CAD build for the part. Positions are in the model's coordinates, mm. A direction names the side the tool comes from. Give positions to 0.01 mm unless a question says otherwise; leave off trailing zeros. Loops run counter-clockwise (first coordinate to the right, second up) from the corner with the lowest first, then second, coordinate; pieces in that order, holes last. Notation, with made-up numbers: M -39.75,-20 L -17.75,-20 A15 cw -17.75,-9 Z; hole C 19,66.25 d10. An arc over 180 degrees is marked long. Answer as CSV lines item,"result".
from build123d import *

# Parameters (mm, degrees)
SKETCH_1_W          = 11
SKETCH_1_H          = 9.5
EXTRUDE_1_DEPTH     = 3
CUT_EXTRUDE_1_DEPTH = 0.5
FILLET_1_R          = 0.7
SKETCH_3_R          = 1.9
EXTRUDE_2_DEPTH     = 0.2
CUT_EXTRUDE_2_DEPTH = 15.783098457
EXTRUDE_3_DEPTH     = 0.2
EXTRUDE_4_DEPTH     = 1
SKETCH_7_R          = 0.75
EXTRUDE_5_DEPTH     = 0.5
SKETCH_8_R          = 0.75
SKETCH_8_R_2        = 2
EXTRUDE_6_DEPTH     = 0.3


with BuildPart() as part:
    # 草图1 → 凸台-拉伸1 (new body)
    with BuildSketch(Plane.XY):
        with Locations((5.5, 4.75)):
            Rectangle(SKETCH_1_W, SKETCH_1_H)
    extrude(amount=EXTRUDE_1_DEPTH)

    # 草图2 → 切除-拉伸1 (cut)
    with BuildSketch(Plane.XY.offset(3)):
        with BuildLine():
            Line((9.028427125, 5.75), (10.33067791, 5.75))
            ThreePointArc((10.33067791, 5.75), (9.020226339, 7.929437592), (6.7, 8.970485754))
            Line((6.7, 8.970485754), (6.7, 7.708039892))
            ThreePointArc((6.7, 7.708039892), (8.130825429, 7.046064713), (9.028427125, 5.75))
        make_face()
        with BuildLine():
            Line((3.371572875, 3.75), (2.06932209, 3.75))
            ThreePointArc((2.06932209, 3.75), (3.379773661, 1.570562408), (5.7, 0.529514246))
            Line((5.7, 0.529514246), (5.7, 1.791960108))
            ThreePointArc((5.7, 1.791960108), (4.269174571, 2.453935287), (3.371572875, 3.75))
        make_face()
        with BuildLine():
            Line((2.06932209, 5.75), (3.371572875, 5.75))
            ThreePointArc((3.371572875, 5.75), (4.269174571, 7.046064713), (5.7, 7.708039892))
            Line((5.7, 7.708039892), (5.7, 8.970485754))
            ThreePointArc((5.7, 8.970485754), (3.379773661, 7.929437592), (2.06932209, 5.75))
        make_face()
        with BuildLine():
            Line((10.33067791, 3.75), (9.028427125, 3.75))
            ThreePointArc((9.028427125, 3.75), (8.130825429, 2.453935287), (6.7, 1.791960108))
            Line((6.7, 1.791960108), (6.7, 0.529514246))
            ThreePointArc((6.7, 0.529514246), (9.020226339, 1.570562408), (10.33067791, 3.75))
        make_face()
        with BuildLine():
            Line((5.7, 7.199489743), (5.7, 6.95))
            Line((5.7, 6.95), (6.7, 6.95))
            Line((6.7, 6.95), (6.7, 7.199489743))
            ThreePointArc((6.7, 7.199489743), (8.7, 4.75), (6.7, 2.300510257))
            Line((6.7, 2.300510257), (6.7, 2.55))
            Line((6.7, 2.55), (5.7, 2.55))
            Line((5.7, 2.55), (5.7, 2.300510257))
            ThreePointArc((5.7, 2.300510257), (3.7, 4.75), (5.7, 7.199489743))
        make_face()
    extrude(amount=-CUT_EXTRUDE_1_DEPTH, mode=Mode.SUBTRACT)

    # 圆角1
    fillet_1_edges = [part.edges().sort_by_distance(p)[0] for p in [
        (0, 0, 1.5),
        (0, 9.5, 1.5),
        (11, 9.5, 1.5),
        (11, 0, 1.5),
    ]]
    fillet(fillet_1_edges, radius=FILLET_1_R)

    # 草图3 → 凸台-拉伸2 (add)
    with BuildSketch(Plane.XY.offset(2.5)):
        with Locations((6.2, 4.75)):
            Circle(SKETCH_3_R)
    extrude(amount=EXTRUDE_2_DEPTH)

    # 草图4 → 切除-拉伸2 (cut, through all)
    with BuildSketch(Plane.XY.offset(2.7)):
        Polygon((6.15, 5.55), (6.25, 5.55), (6.25, 5.25), (7.3, 5.25), (7.3, 4.25), (6.25, 4.25), (6.25, 3.95), (6.15, 3.95), (6.15, 4.25), (5.1, 4.25), (5.1, 4.75), (5.1, 5.25), (6.15, 5.25), align=None)
    extrude(amount=-CUT_EXTRUDE_2_DEPTH, mode=Mode.SUBTRACT)

    # 草图5 → 凸台-拉伸3 (add)
    with BuildSketch(Plane.XY.offset(2.7)):
        with BuildLine():
            Line((5.1, 4.25), (5.1, 5.25))
            Line((5.1, 5.25), (4.366969722, 5.25))
            ThreePointArc((4.366969722, 5.25), (4.3, 4.75), (4.366969722, 4.25))
            Line((4.366969722, 4.25), (5.1, 4.25))
        make_face()
        with BuildLine():
            Line((7.3, 5.25), (8.033030278, 5.25))
            ThreePointArc((8.033030278, 5.25), (8.1, 4.75), (8.033030278, 4.25))
            Line((8.033030278, 4.25), (7.3, 4.25))
            Line((7.3, 4.25), (7.3, 5.25))
        make_face()
    extrude(amount=EXTRUDE_3_DEPTH)

    # 草图6 → 凸台-拉伸4 (add)
    with BuildSketch(Plane.XZ.offset(-4.25)):
        Polygon((5.1, 2.9), (5.1, 3.2), (4.1, 2.9), align=None)
        Polygon((7.3, 2.9), (7.3, 3.2), (8.3, 2.9), align=None)
    extrude(amount=-EXTRUDE_4_DEPTH)

    # 草图7 → 凸台-拉伸5 (add)
    with BuildSketch(Plane(origin=(0, 0, 0), x_dir=(-1, 0, 0), z_dir=(0, 0, -1))):
        with Locations((-10, 8.5)):
            Circle(SKETCH_7_R)
        with Locations((-3, 8.5)):
            Circle(SKETCH_7_R)
        with Locations((-3, 1)):
            Circle(SKETCH_7_R)
        with Locations((-10, 1)):
            Circle(SKETCH_7_R)
    extrude(amount=EXTRUDE_5_DEPTH)

    # 草图8 → 凸台-拉伸6 (add)
    with BuildSketch(Plane(origin=(0, 0, 0), x_dir=(-1, 0, 0), z_dir=(0, 0, -1))):
        with BuildLine():
            Line((-2.05, 0.7), (-2.05, 2.75))
            Line((-2.05, 2.75), (-2.55, 2.75))
            Line((-2.55, 2.75), (-2.55, 4.75))
            Line((-2.55, 4.75), (-2.55, 6.75))
            Line((-2.55, 6.75), (-2.05, 6.75))
            Line((-2.05, 6.75), (-2.05, 8.8))
            ThreePointArc((-2.05, 8.8), (-2.240380592, 9.259619408), (-2.7, 9.45))
            Line((-2.7, 9.45), (-4.5, 9.45))
            Line((-4.5, 9.45), (-4.5, 8.95))
            Line((-4.5, 8.95), (-6.5, 8.95))
            Line((-6.5, 8.95), (-8.5, 8.95))
            Line((-8.5, 8.95), (-8.5, 9.45))
            Line((-8.5, 9.45), (-10.3, 9.45))
            ThreePointArc((-10.3, 9.45), (-10.759619408, 9.259619408), (-10.95, 8.8))
            Line((-10.95, 8.8), (-10.95, 6.75))
            Line((-10.95, 6.75), (-10.45, 6.75))
            Line((-10.45, 6.75), (-10.45, 4.75))
            Line((-10.45, 4.75), (-10.45, 2.75))
            Line((-10.45, 2.75), (-10.95, 2.75))
            Line((-10.95, 2.75), (-10.95, 0.7))
            ThreePointArc((-10.95, 0.7), (-10.759619408, 0.240380592), (-10.3, 0.05))
            Line((-10.3, 0.05), (-8.5, 0.05))
            Line((-8.5, 0.05), (-8.5, 0.55))
            Line((-8.5, 0.55), (-7.5, 0.55))
            Line((-7.5, 0.55), (-6.5, 0.55))
            Line((-6.5, 0.55), (-4.5, 0.55))
            Line((-4.5, 0.55), (-4.5, 0.05))
            Line((-4.5, 0.05), (-2.7, 0.05))
            ThreePointArc((-2.7, 0.05), (-2.240380592, 0.240380592), (-2.05, 0.7))
        make_face()
        with Locations(Location((-10, 8.5, 0), (0, 0, 180))):
            Circle(SKETCH_8_R, mode=Mode.SUBTRACT)
        with Locations(Location((-3, 8.5, 0), (0, 0, 180))):
            Circle(SKETCH_8_R, mode=Mode.SUBTRACT)
        with Locations(Location((-10, 1, 0), (0, 0, 180))):
            Circle(SKETCH_8_R, mode=Mode.SUBTRACT)
        with Locations(Location((-3, 1, 0), (0, 0, 180))):
            Circle(SKETCH_8_R, mode=Mode.SUBTRACT)
        with Locations((-6.2, 4.75)):
            Circle(SKETCH_8_R_2, mode=Mode.SUBTRACT)
    extrude(amount=EXTRUDE_6_DEPTH)


solid = part.part
1) Band-saw the part on B-B on z = 0.9. Give the cut face in (x, y).
Answer below:
outline,"M 0,0.7 A0.7 ccw 0.7,0 L 10.3,0 A0.7 ccw 11,0.7 L 11,8.8 A0.7 ccw 10.3,9.5 L 0.7,9.5 A0.7 ccw 0,8.8 Z; hole M 5.1,4.25 L 6.15,4.25 L 6.15,3.95 L 6.25,3.95 L 6.25,4.25 L 7.3,4.25 L 7.3,5.25 L 6.25,5.25 L 6.25,5.55 L 6.15,5.55 L 6.15,5.25 L 5.1,5.25 Z"
2) Flat gauge pins, fed straight in: pin 1 (1 mm diameter, centred on x = 4.5, y = 2, fed in from +Z); pin 2 (4.5 mm diameter, centred on x = 8, y = 5, fed in from -Z). Where does each tip first touch, or does it go through?
Answer below:
pin 1,"stops at z = 3"
pin 2,"stops at z = -0.3"
3) Band-saw the part on D-D on x = 3. Give the cut face in (y, z).
Answer below:
outline,"M 0,0 L 0.05,0 L 0.05,-0.3 L 0.25,-0.3 L 0.25,-0.5 L 1.75,-0.5 L 1.75,-0.3 L 7.75,-0.3 L 7.75,-0.5 L 9.25,-0.5 L 9.25,-0.3 L 9.45,-0.3 L 9.45,0 L 9.5,0 L 9.5,3 L 7.55,3 L 7.55,2.5 L 5.75,2.5 L 5.75,3 L 3.75,3 L 3.75,2.5 L 1.95,2.5 L 1.95,3 L 0,3 Z"
4) Which spindle directions (+Z, -Z, +X, -X, +Y, -Y) get a long thin tool onto all of the face, cutting with end or side? Do faces 4 (the face through (6, 4, 0)), 5 (the face through (6, 4, 2.7)), 6 (the face through (5.1, 5, 2)). Say none if no direction does.
Answer below:
face 4,"-Z"
face 5,"+Z"
face 6,"+Z, -Z"
5) Band-saw the part on C-C on y = 8.5. Give the cut face in (x, z), and give its area (3 significant figures).
Answer below:
outline,"M 0,0 L 2.05,0 L 2.05,-0.3 L 2.25,-0.3 L 2.25,-0.5 L 3.75,-0.5 L 3.75,-0.3 L 9.25,-0.3 L 9.25,-0.5 L 10.75,-0.5 L 10.75,-0.3 L 10.95,-0.3 L 10.95,0 L 11,0 L 11,3 L 8.2,3 L 8.2,2.5 L 6.7,2.5 L 6.7,3 L 5.7,3 L 5.7,2.5 L 4.2,2.5 L 4.2,3 L 0,3 Z"
area,"34.8 mm^2"
6) Band-saw the part on A-A on y = 4.75. Give the cut face in (x, z), and give its area (3 significant figures).
Answer below:
outline,"M 0,0 L 2.55,0 L 2.55,-0.3 L 4.2,-0.3 L 4.2,0 L 5.1,0 L 5.1,3.2 L 4.1,2.9 L 4.3,2.9 L 4.3,2.5 L 3.7,2.5 L 3.7,3 L 0,3 Z; M 7.3,0 L 8.2,0 L 8.2,-0.3 L 10.45,-0.3 L 10.45,0 L 11,0 L 11,3 L 8.7,3 L 8.7,2.5 L 8.1,2.5 L 8.1,2.9 L 8.3,2.9 L 7.3,3.2 Z"
area,"27.1 mm^2"
7) Drill centre lines: line 1 (Y direction, x = 6.2, z = -0.15); line 2 (X direction, y = 8, z = 2.85); line 3 (X direction, y = 2.25, z = 2.6). Where is each one in solid material? Low to high. Write a range as from..to.
Answer below:
line 1,"y = 0.55..2.75, 6.75..8.95"
line 2,"x = 0..3.46, 5.7..6.7, 8.94..11"
line 3,"x = 0..2.76, 4.54..7.86, 9.64..11"
8) Mould opens along Y. For faces 1 (the face through (5, 9.5, 1)), 2 (the face through (7, 4.25, 1)), 3 (the face through (0, 5, 1)) say: +Y half, -Y half, draft (parallel to the pull), parting line (faces both ways), or undercut.
Answer below:
face 1,"+Y half"
face 2,"undercut"
face 3,"draft"
